from build123d import *

# Parameters (mm, degrees)
F1_DEPTH = 8
F0_W     = 1.5
F0_H     = 2
F2_DEPTH = 7
F0_W_2   = 2.5
F3_DEPTH = 2


with BuildPart() as f1:
    # F0 (on Top) → F1 (new body)
    with BuildSketch(Plane.XY):
        Polygon((-2.5, 2), (0, 2), (0, 3.5), (-4, 3.5), (-4, 2), align=None)
    extrude(amount=F1_DEPTH)

    # F0 (on Top) → F2 (join)
    with BuildSketch(Plane.XY):
        with Locations((-3.25, 1)):
            Rectangle(F0_W, F0_H)
    extrude(amount=F2_DEPTH)

    # F0 (on Top) → F3 (join)
    with BuildSketch(Plane.XY):
        with Locations((-1.25, 1)):
            Rectangle(F0_W_2, F0_H)
    extrude(amount=F3_DEPTH)


solid = f1.part
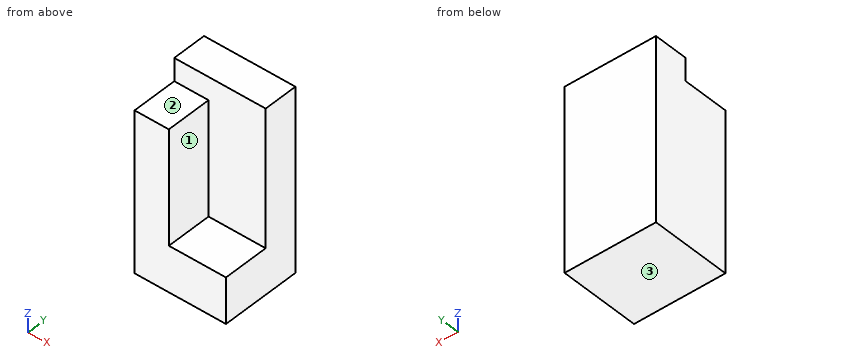
Model file for the job. Use its own axes, mm. Face numbers are marked on the shaded views. A direction names the side the tool comes from. Give positions to 0.01 mm unless a question says otherwise; leave off trailing zeros. Loops run counter-clockwise (first coordinate to the right, second up) from the corner with the lowest first, then second, coordinate; pieces in that order, holes last.
1) Wall check: line 1 (Z direction, x = -1.75, y = 1.9); line 2 (Z direction, x = -2.9, y = 0.4); line 3 (Y direction, x = -1.65, z = 7). Give the ranges that are in metal, low to high.
2) Flat gauge pins, fed straight in: pin 1 Ø2 at (y, z) = (2, 4) entering from +X; pin 2 Ø0.8 at (x, y) = (-3.5, 0.5) entering from +Z; pin 3 Ø1 at (x, y) = (-1.5, 1) entering from +Z. Where does each tip first touch, or does it go through?
3) Saw through at A-A (x = -3.3). Write the cut outline in (y, z), plus the area to 3 significant figures.
4) Saw through at B-B (z = 2.5). Write the cut outline in (x, y).
5) Tool access for the marked faces 1, 2 and 3: list every direction of +Z, -Z, +X, -X, +Y, -Y with a clear straight run to the whole face (end or side of a thin tool).
Answer block:
1. line 1: z = 0 to 2
1. line 2: z = 0 to 7
1. line 3: y = 2 to 3.5
2. pin 1: stops at x = 0
2. pin 2: stops at z = 7
2. pin 3: stops at z = 2
3. outline: (0, 0) - (3.5, 0) - (3.5, 8) - (2, 8) - (2, 7) - (0, 7) - close
3. area: 26.0 mm2
4. outline: (-4, 0) - (-2.5, 0) - (-2.5, 2) - (0, 2) - (0, 3.5) - (-4, 3.5) - close
5. face 1: +Z, +X, -Y
5. face 2: +Z, +X, -X, -Y
5. face 3: -Z, +X, -X, +Y, -Y
